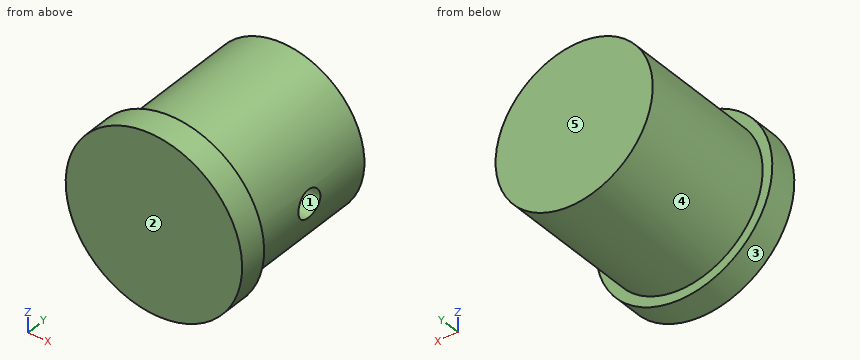
```python
from build123d import *

# Parameters (mm, degrees)
F6_D     = 2
F6_DEPTH = 5.7
F6_TIP   = 0.600860619


# Not quite as in the source:
# - a feature names something its author has since deleted; it is built from what else it names


with BuildPart() as f3:
    # F2 (on Right) → F3 (revolve)
    with BuildSketch(Plane.YZ):
        Polygon((0, 0), (12, 0), (12, 5.7), (2, 5.7), (2, 6.4), (0, 6.4), align=None)
    revolve(axis=Axis((0, 5.7350749573, 0), (0, -1, 0)))

    # F6
    with Locations(Plane.YZ.offset(5.7)):
        with Locations((7, 0)):
            Hole(F6_D / 2, depth=F6_DEPTH)
            with Locations((0, 0, -(F6_DEPTH + F6_TIP / 2))):  # 118° drill point
                Cone(0, F6_D / 2, F6_TIP, mode=Mode.SUBTRACT)


solid = f3.part
```
Part model, mm, in its own coordinate system. Face numbers are marked on the shaded views. A direction names the side the tool comes from. Round coordinates to 2 decimals unless told otherwise and drop trailing zeros. Write each loop counter-clockwise with the first axis right and the second up, starting at its lowest first coordinate (ties: lowest second). Pieces come first, ordered by that corner, then holes. Notation, with made-up numbers: (-35, 82.25) -> (-5, 82.25) arc R22 cw to (-5, 93.25) -> close; hole circle Ø11 at (-26.5, 1.5). An arc over 180 degrees is marked (long way). Return JSON: item names as keys, results as strings. Group by question number.
Q1. Saw through at C-C on x = -2.25. Write the cut outline in (y, z), plus the area to 3 significant figures.
Q2. Saw through at B-B on z = -2.75. Write the cut outline in (x, y).
Q3. Saw through at D-D on y = 5.75. Write the cut outline in (x, z).
Q4. Which spindle directions (+Z, -Z, +X, -X, +Y, -Y) get a long thin tool onto all of the face, cutting with end or side? Do the marked faces 4 and 5. Say none if no direction does.
Q5. Saw through at A-A on x = 3. Write the cut outline in (y, z).
Q6. Probe L1, parallel to Y at x = 3.1, z = 0; L2, parallel to Y at x = -4.75, z = 3.25; L3, parallel to Z at x = 2.5, y = 7.25. List the from-to ranges inside material, lowest first. Write a range as [from, to].
Q7. Pin check, flat tips, straight feed: pin 1 (6 mm diameter, centred on y = 5.5, z = -4.5, fed in from -X); pin 2 (1.5 mm diameter, centred on x = 3, y = 10.5, fed in from +Z); pin 3 (3 mm diameter, centred on y = 7.5, z = -1.5, fed in from -X). Stop position of each tip, or through.
Q8. Mould opens along Y. For the marked faces 1, 2 and 3 say: pulls with the +Y half, pulls with the -Y half, needs draft (parallel to the pull), parting line crosses it, or undercut.
Answer:
{
 "1": {"outline": "(0, -5.99) -> (2, -5.99) -> (2, -5.24) -> (12, -5.24) -> (12, 5.24) -> (2, 5.24) -> (2, 5.99) -> (0, 5.99) -> close", "area": "129 mm2"},
 "2": {"outline": "(-5.78, 0) -> (5.78, 0) -> (5.78, 2) -> (4.99, 2) -> (4.99, 12) -> (-4.99, 12) -> (-4.99, 2) -> (-5.78, 2) -> close"},
 "3": {"outline": "circle Ø11.4 at (0, 0)"},
 "4": {"face 4": "+Y", "face 5": "+Z, -Z, +X, -X, +Y"},
 "5": {"outline": "(0, -5.65) -> (2, -5.65) -> (2, -4.85) -> (12, -4.85) -> (12, 4.85) -> (2, 4.85) -> (2, 5.65) -> (0, 5.65) -> close; hole circle Ø2 at (7, 0)"},
 "6": {"L1": "[0, 6], [8, 12]", "L2": "[0, 2]", "L3": "[-5.12, -0.97], [0.97, 5.12]"},
 "7": {"pin 1": "x = -5.5", "pin 2": "z = 5.24", "pin 3": "x = -5.7"},
 "8": {"face 1": "undercut", "face 2": "pulls with the -Y half", "face 3": "needs draft"}
}
